Input: part model. Units: mm. Frame: model coordinates. A direction names the side the tool comes from. Coordinates: 2 decimals unless noted, no trailing zeros. Loops run counter-clockwise (first coordinate to the right, second up) from the corner with the lowest first, then second, coordinate; pieces in that order, holes last.
(1) Contact query for flat-ended pins moving along their axis: P1, Ø10, axis at x = 103.5, y = -7, coming from the +Z side; P2, Ø1.5, axis at y = -2.5, z = 3, coming from the +X side; P3, Ø1, axis at x = -51.5, y = 12.5, coming from the +Z side. Output: stop coordinate, or through.
(2) Section B-B, the plane x = 19.5. Return loops of the section in (y, z), then the cut area to 3 significant figures.
(3) Section A-A, the plane x = 77. Return loops of the section in (y, z).
(4) Line query: L1, parallel to Y at x = -33, z = 5; L2, parallel to X at y = -1, z = 3.25; L3, parallel to Z at x = 61, y = 8.5. Output: solid intervals per line, ascending.
(5) Mould query, pull axis Y, two halves, no side actions, for faces 1 (the face through (-1, 0, 2)), 2 (the face through (126.46, -0.74, 6.68)), 3 (the face through (27, 0, 0)), 4 (the face through (125.142, 0.715, 5.479)). Classes: released by +Y, released by -Y, zero draft, split by the parting line, or undercut.
(6) Set-up query: faces 5 (the face through (10, 35.5, 2)), 6 (the face through (9, 32.5, 4)). Return all of +Z, -Z, +X, -X, +Y, -Y with unobstructed straight access to the full face (end or side cutting, diameter ignored); none if empty.
```python
from build123d import *

# Parameters (mm, degrees)
F0_W     = 145.3
F0_H     = 65
F1_DEPTH = 2
F0_W_2   = 20
F3_DEPTH = 4
F4_DEPTH = 2
F0_H_2   = 3
F5_DEPTH = 7
F6_DEPTH = 7
F7_SIZE  = 1.99999


# Not quite as in the source:
# - a fillet or chamfer is up to 0.001 mm smaller than in the source, because OpenCascade refuses the exact size


with BuildPart() as f1:
    # F0 (on Top) → F1 (new body)
    with BuildSketch(Plane.XY):
        Rectangle(F0_W, F0_H)
    extrude(amount=F1_DEPTH)

    # F0 (on Top) → F3 (join)
    with BuildSketch(Plane.XY):
        with Locations((82.65, 0)):
            Rectangle(F0_W_2, F0_H)
        with BuildLine():
            ThreePointArc((92.65, -32.5), (125.15, 0), (92.65, 32.5))
            Line((92.65, 32.5), (92.65, -32.5))
        make_face()
    extrude(amount=F3_DEPTH)

    # F2 (on face) → F4 (join)
    with BuildSketch(Plane.XY.offset(2)):
        with BuildLine():
            ThreePointArc((47.65, 32.5), (65.6769816336, 20.5015243336), (72.65, 0))
            Line((72.65, 0), (72.65, 32.5))
            Line((72.65, 32.5), (47.65, 32.5))
        make_face()
        with BuildLine():
            ThreePointArc((72.65, 0), (65.6769816336, -20.5015243336), (47.65, -32.5))
            Line((47.65, -32.5), (72.65, -32.5))
            Line((72.65, -32.5), (72.65, 0))
        make_face()
    extrude(amount=F4_DEPTH)

    # F0 (on Top) → F5 (join)
    with BuildSketch(Plane.XY):
        with BuildLine():
            Line((92.65, 35.5), (92.65, 32.5))
            ThreePointArc((92.65, 32.5), (125.15, 0), (92.65, -32.5))
            Line((92.65, -32.5), (92.65, -35.5))
            ThreePointArc((92.65, -35.5), (128.15, 0), (92.65, 35.5))
        make_face()
        with Locations((82.65, -34)):
            Rectangle(F0_W_2, F0_H_2)
        with Locations((82.65, 34)):
            Rectangle(F0_W_2, F0_H_2)
    extrude(amount=F5_DEPTH)

    # F0 (on Top) → F6 (join)
    with BuildSketch(Plane.XY):
        with Locations((0, -34)):
            Rectangle(F0_W, F0_H_2)
        with Locations((0, 34)):
            Rectangle(F0_W, F0_H_2)
    extrude(amount=F6_DEPTH)

    # F7 (size 2 in the source; OpenCascade refuses exactly that, so slightly less here)
    f7_edges = [f1.edges().sort_by_distance(p)[0] for p in [
        (-72.65, 35.5, 3.5),
        (-72.65, -35.5, 3.5),
        (-72.65, -34, 7),
        (-72.65, 34, 7),
        (-72.65, 0, 0),
        (10, 35.5, 7),
    ]]
    chamfer(f7_edges, length=F7_SIZE)


solid = f1.part
```
Report:
1. P1: stops at z = 4
1. P2: stops at x = 128.11
1. P3: stops at z = 2
2. outline: (-35.5, 0) - (35.5, 0) - (35.5, 5) - (33.5, 7) - (32.5, 7) - (32.5, 2) - (-32.5, 2) - (-32.5, 7) - (-33.5, 7) - (-35.5, 5) - close
2. area: 168 mm2
3. outline: (-35.5, 0) - (35.5, 0) - (35.5, 5) - (33.5, 7) - (32.5, 7) - (32.5, 4) - (-32.5, 4) - (-32.5, 7) - (-33.5, 7) - (-35.5, 5) - close
4. L1: y = -35.5 to -32.5, 32.5 to 35.5
4. L2: x = 72.64 to 128.14
4. L3: z = 0 to 2
5. face 1: undercut
5. face 2: split by the parting line
5. face 3: zero draft
5. face 4: undercut
6. face 5: +Z, -Z, +X, -X, +Y
6. face 6: +Z, -X
